Design review of the part built by this model. Coordinates are the model's own, in mm. A direction names the side the tool comes from. Coordinates: 2 decimals unless noted, no trailing zeros. Write each loop counter-clockwise with the first axis right and the second up, starting at its lowest first coordinate (ties: lowest second). Pieces come first, ordered by that corner, then holes.
Q1. Insertion check: pin 1 (0.6 mm diameter, centred on x = 15, z = 1, fed in from +Y); pin 2 (0.6 mm diameter, centred on y = 25, z = 1, fed in from +X). Each pin has a flat end and moves straight along its axis. Give the tip position at first contact, or say it passes through.
Q2. Mouldability with a two-part tool opening along Y and no side actions: class faces 3 (the cylindrical face through (-10.2, 7.1, 1)), 4 (the flat face through (-8, 15, 0)), 5 (the cylindrical face through (6.711, 6.804, 1.014)) as pulls with the +Y half, pulls with the -Y half, needs draft (parallel to the pull), parting line crosses it, or undercut.
Q3. Take a section at B-B (x = -8.5). Give the boundary of the cut face in (y, z), and give its area (3 significant figures).
Q4. Take a section at A-A (y = 35). Give the boundary of the cut face in (x, z).
Q5. Take a section at D-D (y = 17). Give the boundary of the cut face in (x, z), and give its area (3 significant figures).
Q6. Take a section at C-C (z = 1.1). Give the boundary of the cut face in (x, y), and give its area (3 significant figures).
Q7. Machinability: for faces 1 (the flat face through (-8, 15, 2)), 2 (the flat face through (15, 5, 1)), which of the approach directions +Z, -Z, +X, -X, +Y, -Y give a long, thin tool a straight path to every point of the face, cutting with its end or side? Answer none if there is none.
Q8. For probe 1 along Y at (x, z) = (0, 1.5); probe 2 along Y at (x, z) = (15, 0.7); probe 3 along Y at (x, z) = (-30, 0.55), list the stretches that pass through material, from the lowest coordinate up.
```python
from build123d import *

# Parameters (mm, degrees)
SKETCH_1_R          = 1.5
EXTRUDE_1_DEPTH     = 2
CUT_EXTRUDE_1_DEPTH = 10
FILLET_1_R          = 1


with BuildPart() as part:
    # 草图1 → 凸台-拉伸1 (new body)
    with BuildSketch(Plane.XY):
        Polygon((-5, 45), (-35, 5), (-35, -4), (20, -4), (20, 5), (5, 45), align=None)
        with Locations((-30, 0)):
            Circle(SKETCH_1_R, mode=Mode.SUBTRACT)
        with Locations((-15, 0)):
            Circle(SKETCH_1_R, mode=Mode.SUBTRACT)
        with Locations((-9, 8)):
            Circle(SKETCH_1_R, mode=Mode.SUBTRACT)
        with Locations((15, 0)):
            Circle(SKETCH_1_R, mode=Mode.SUBTRACT)
        with Locations((0, 20)):
            Circle(SKETCH_1_R, mode=Mode.SUBTRACT)
        with Locations((0, 35)):
            Circle(SKETCH_1_R, mode=Mode.SUBTRACT)
    extrude(amount=EXTRUDE_1_DEPTH)

    # 草图2 → 切除-拉伸1 (cut)
    with BuildSketch(Plane.XY.offset(2)):
        with BuildLine():
            Line((5, 45), (5, 11))
            ThreePointArc((5, 11), (6.757359313, 6.757359313), (11, 5))
            Line((11, 5), (20, 5))
            Line((20, 5), (5, 45))
        make_face()
    extrude(amount=-CUT_EXTRUDE_1_DEPTH, mode=Mode.SUBTRACT)

    # 圆角1
    fillet_1_edges = [part.edges().sort_by_distance(p)[0] for p in [
        (20, -4, 1),
        (-35, -4, 1),
        (-35, 5, 1),
        (-5, 45, 1),
        (5, 45, 1),
        (20, 5, 1),
    ]]
    fillet(fillet_1_edges, radius=FILLET_1_R)


solid = part.part
```
Response:
1. pin 1: stops at y = 5
1. pin 2: stops at x = 5
2. face 3: undercut
2. face 4: needs draft
2. face 5: pulls with the +Y half
3. outline: (-4, 0) - (6.59, 0) - (6.59, 2) - (-4, 2) - close; (9.41, 0) - (40.33, 0) - (40.33, 2) - (9.41, 2) - close
3. area: 83.0 mm2
4. outline: (-12.5, 0) - (-1.5, 0) - (-1.5, 2) - (-12.5, 2) - close; (1.5, 0) - (5, 0) - (5, 2) - (1.5, 2) - close
5. outline: (-26, 0) - (5, 0) - (5, 2) - (-26, 2) - close
5. area: 62.0 mm2
6. outline: (-35, -3) arc R1 ccw to (-34, -4) - (19, -4) arc R1 ccw to (20, -3) - (20, 4) arc R1 ccw to (19, 5) - (11, 5) arc R6 cw to (5, 11) - (5, 44) arc R1 ccw to (4, 45) - (-4.5, 45) arc R1 ccw to (-5.3, 44.6) - (-34.8, 5.27) arc R1 ccw to (-35, 4.67) - close; hole circle Ø3 at (-30, 0); hole circle Ø3 at (-15, 0); hole circle Ø3 at (-9, 8); hole circle Ø3 at (0, 20); hole circle Ø3 at (0, 35); hole circle Ø3 at (15, 0)
6. area: 1,460 mm2
7. face 1: +Z, +X, -X, +Y, -Y
7. face 2: +Z, -Z, +X, +Y
8. probe 1: y = -4 to 18.5, 21.5 to 33.5, 36.5 to 45
8. probe 2: y = -4 to -1.5, 1.5 to 5
8. probe 3: y = -4 to -1.5, 1.5 to 11.67
